The listing builds one solid part. Answer for the finished solid, in the listing's coordinates (mm). Face numbers are marked on the shaded views. A direction names the side the tool comes from. Round coordinates to 2 decimals unless told otherwise and drop trailing zeros. Write each loop counter-clockwise with the first axis right and the second up, starting at its lowest first coordinate (ties: lowest second). Pieces come first, ordered by that corner, then holes. Notation, with made-up numbers: (-9, 47.25) - (34, 47.25) arc R25 ccw to (34, 68.25) - close; hole circle Ø3 at (7, 89). An arc over 180 degrees is marked (long way). Use a Markdown table: item, result. Add a question column.
1) A cutting plane is placed at A-A (z = 0). Give the vertices of the cut face in (x, y).
2) A tool of negligible diameter and unlimited length cuts with its end or side. For the marked faces 4 and 5, from which of +Z, -Z, +X, -X, +Y, -Y can it reach the whole face along a straight path? Write none if from no direction.
3) A cutting plane is placed at C-C (x = 0.75). Give the vertices of the cut face in (y, z) (1 decimal).
4) A cutting plane is placed at B-B (y = 8.5). Give the vertices of the cut face in (x, z).
5) Find the intervals of material crossed by probe 1 along Y at (x, z) = (-3.7, 0); probe 2 along Y at (x, z) = (-1.5, 0); probe 3 along X at (y, z) = (13, -4.5), in increasing order. Write a range as from..to.
6) Determine the mould class of the marked faces 1, 2 and 3 for opening direction Z: +Z half, -Z half, draft (parallel to the pull), parting line (faces both ways), or undercut.
7) Each of these flat-tipped pins is pushed along its axis until it touches: P1, Ø4, axis at x = 2.5, z = -2, coming from the -Y side; P2, Ø1, axis at x = -1.5, y = 13, coming from the -Z side; P3, Ø1.5, axis at x = 3, z = -8, coming from the -Y side. Where does it stop, or does it pass through?
8) A cutting plane is placed at D-D (z = -8.5). Give the vertices of the cut face in (x, y).
```python
from build123d import *

# Parameters (mm, degrees)
BODY_MOVE_COPY1_ANGLE = 90


with BuildPart() as part:
    # Sketch5 → Revolve1 (revolve)
    with BuildSketch(Plane.XY, mode=Mode.PRIVATE) as revolve1_sk:
        Polygon((6.8707, 7.9502), (6.8707, 0), (14.2875, 0), (14.2875, 6.35), (15.5575, 6.35), (15.5575, 7.9502), (12.6619, 7.9502), (12.6619, 7.3152), (9.7663, 7.3152), (9.7663, 7.9502), align=None)
    revolve(revolve1_sk.sketch.rotate(Axis((0, 0, 0), (0, 1, 0)), 90), axis=Axis((0, 0, 0), (0, 1, 0)))


with BuildPart() as part_1:
    # Body-Move/Copy1: moved
    add(part.part.rotate(Axis((0, 3.9751, 0), (0, 0, 1)), BODY_MOVE_COPY1_ANGLE))


solid = part_1.part
```
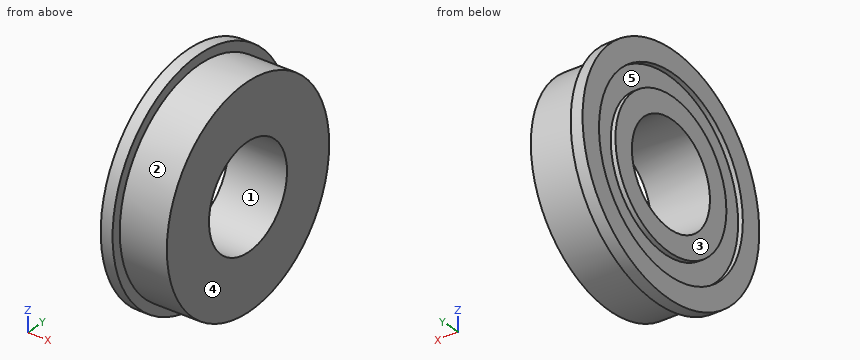
Entries:
| question | item | result |
|---|---|---|
| 1 | outline | (-3.98, -11.58) - (-2.37, -11.58) - (-2.37, -10.31) - (3.98, -10.31) - (3.98, -2.9) - (-3.98, -2.9) - (-3.98, -5.79) - (-3.34, -5.79) - (-3.34, -8.69) - (-3.98, -8.69) - close; (-3.98, 10.85) - (3.98, 10.85) - (3.98, 18.26) - (-2.37, 18.26) - (-2.37, 19.53) - (-3.98, 19.53) - (-3.98, 16.64) - (-3.34, 16.64) - (-3.34, 13.74) - (-3.98, 13.74) - close |
| 2 | face 4 | +Z, -Z, +X, +Y, -Y |
| 2 | face 5 | -X |
| 3 | outline | circle Ø28.6 at (4, 0); hole circle Ø13.7 at (4, 0) |
| 4 | outline | (-3.98, -14.88) - (-2.37, -14.88) - (-2.37, -13.55) - (3.98, -13.55) - (3.98, -5.17) - (-3.98, -5.17) - (-3.98, -8.65) - (-3.34, -8.65) - (-3.34, -11.83) - (-3.98, -11.83) - close; (-3.98, 5.17) - (3.98, 5.17) - (3.98, 13.55) - (-2.37, 13.55) - (-2.37, 14.88) - (-3.98, 14.88) - (-3.98, 11.83) - (-3.34, 11.83) - (-3.34, 8.65) - (-3.98, 8.65) - close |
| 5 | probe 1 | y = -11.58..-8.69, -5.79..-2.9, 10.85..13.74, 16.64..19.53 |
| 5 | probe 2 | y = -10.31..-2.9, 10.85..18.26 |
| 5 | probe 3 | x = -3.34..3.98 |
| 6 | face 1 | undercut |
| 6 | face 2 | parting line |
| 6 | face 3 | draft |
| 7 | P1 | stops at y = -10.31 |
| 7 | P2 | stops at z = -11.47 |
| 7 | P3 | stops at y = -8.34 |
| 8 | outline | (-3.98, -9.06) - (-2.37, -9.06) - (-2.37, -7.51) - (3.98, -7.51) - (3.98, 15.46) - (-2.37, 15.46) - (-2.37, 17.01) - (-3.98, 17.01) - (-3.98, 13.36) - (-3.34, 13.36) - (-3.34, 8.78) - (-3.98, 8.78) - (-3.98, -0.83) - (-3.34, -0.83) - (-3.34, -5.41) - (-3.98, -5.41) - close |
